from build123d import *

# Parameters (mm, degrees)
CORNERBOSS_EXTRUDE1_DEPTH               = 20
SHELL4_T                                = -3
PADSKETCH2_R                            = 12
PADBOSS_EXTRUDE2_DEPTH                  = 10
STEPPERSHAFTHOLECUTSKETCH3_R            = 5.1
STEPPERSHAFTHOLECUT_EXTRUDE1_DEPTH      = 288.430740571
THREADEDNUTMOUNTHOLESSKETCH4_R          = 2
THREADEDNUTMOUNTHOLESCUT_EXTRUDE2_DEPTH = 10
BRPEGHOLESKETCH1_W                      = 10
BRPEGHOLESKETCH1_H                      = 14
BRPEGHOLECUT_EXTRUDE1_DEPTH             = 3
TOPPEGSKETCH2_W                         = 9.8
TOPPEGSKETCH2_H                         = 13.9
TOPPEGBOSS_EXTRUDE1_DEPTH               = 3
TOPPEGCAPSKETCH3_W                      = 16
TOPPEGCAPSKETCH3_H                      = 17
TOPPEGCAPBOSS_EXTRUDE2_DEPTH            = 3.1
CENTERPEGHOLECUTSKETCH1_W               = 10
CENTERPEGHOLECUTSKETCH1_H               = 14
CENTERPEGHOLECUT_EXTRUDE1_DEPTH         = 3


with BuildPart() as part:
    # CornerrSketch1 → CornerBoss-Extrude1 (new body)
    with BuildSketch(Plane(origin=(0, 0, 0), x_dir=(1, 0, 0), z_dir=(0, 1, 0))):
        with BuildLine():
            Line((0, 195.825), (70, 195.825))
            Line((70, 195.825), (70, 125.825))
            Line((70, 125.825), (210, 125.825))
            Line((210, 125.825), (210, 45.825))
            Line((210, 45.825), (34, 45.825))
            Line((34, 45.825), (34, 0))
            ThreePointArc((34, 0), (17, -17), (0, 0))
            Line((0, 0), (0, 195.825))
        make_face()
    extrude(amount=CORNERBOSS_EXTRUDE1_DEPTH)

    # Shell4
    shell4_openings = [part.faces().sort_by_distance(p)[0] for p in [
        (83.067785517, 0, -95.408443826),
    ]]
    offset(amount=SHELL4_T, openings=shell4_openings, kind=Kind.INTERSECTION)

    # PadSketch2 → PadBoss-Extrude2 (add)
    with BuildSketch(Plane.XZ.offset(-17)):
        with Locations(Location((17, 0, 0), (0, 0, 90))):
            Circle(PADSKETCH2_R)
    extrude(amount=PADBOSS_EXTRUDE2_DEPTH)

    # StepperShaftHoleCutSketch3 → StepperShaftHoleCut-Extrude1 (cut, through all)
    with BuildSketch(Plane.XZ.offset(-7)):
        with Locations(Location((17, 0, 0), (0, 0, 270))):
            Circle(STEPPERSHAFTHOLECUTSKETCH3_R)
    extrude(amount=-STEPPERSHAFTHOLECUT_EXTRUDE1_DEPTH, mode=Mode.SUBTRACT)

    # ThreadedNutMountHolesSketch4 → ThreadedNutMountHolesCut-Extrude2 (cut)
    with BuildSketch(Plane(origin=(0, 7, 0), x_dir=(-1, 0, 0), z_dir=(0, -1, 0))):
        with Locations(Location((-17, 8, 0), (0, 0, 90))):
            Circle(THREADEDNUTMOUNTHOLESSKETCH4_R)
        with Locations(Location((-17, -8, 0), (0, 0, 90))):
            Circle(THREADEDNUTMOUNTHOLESSKETCH4_R)
        with Locations(Location((-25, 0, 0), (0, 0, 90))):
            Circle(THREADEDNUTMOUNTHOLESSKETCH4_R)
        with Locations(Location((-9, 0, 0), (0, 0, 90))):
            Circle(THREADEDNUTMOUNTHOLESSKETCH4_R)
    extrude(amount=-THREADEDNUTMOUNTHOLESCUT_EXTRUDE2_DEPTH, mode=Mode.SUBTRACT)

    # BRPegHoleSketch1 → BRPegHoleCut-Extrude1 (cut)
    with BuildSketch(Plane(origin=(210, 0, 0), x_dir=(0, 0, -1), z_dir=(1, 0, 0))):
        with Locations((60.825, 7)):
            Rectangle(BRPEGHOLESKETCH1_W, BRPEGHOLESKETCH1_H)
    extrude(amount=-BRPEGHOLECUT_EXTRUDE1_DEPTH, mode=Mode.SUBTRACT)

    # TopPegSketch2 → TopPegBoss-Extrude1 (add)
    with BuildSketch(Plane(origin=(0, 0, -195.825), x_dir=(-1, 0, 0), z_dir=(0, 0, -1))):
        with Locations((-15, 6.95)):
            Rectangle(TOPPEGSKETCH2_W, TOPPEGSKETCH2_H)
    extrude(amount=TOPPEGBOSS_EXTRUDE1_DEPTH)

    # TopPegCapSketch3 → TopPegCapBoss-Extrude2 (add)
    with BuildSketch(Plane(origin=(0, 0, -198.825), x_dir=(-1, 0, 0), z_dir=(0, 0, -1))):
        with Locations((-14.9, 8.5)):
            Rectangle(TOPPEGCAPSKETCH3_W, TOPPEGCAPSKETCH3_H)
    extrude(amount=TOPPEGCAPBOSS_EXTRUDE2_DEPTH)

    # CenterPegHoleCutSketch1 → CenterPegHoleCut-Extrude1 (cut)
    with BuildSketch(Plane(origin=(0, 0, -125.825), x_dir=(-1, 0, 0), z_dir=(0, 0, -1))):
        with Locations((-175, 7)):
            Rectangle(CENTERPEGHOLECUTSKETCH1_W, CENTERPEGHOLECUTSKETCH1_H)
    extrude(amount=-CENTERPEGHOLECUT_EXTRUDE1_DEPTH, mode=Mode.SUBTRACT)


solid = part.part
Design review of the part built by this model. Coordinates are the model's own, in mm. A direction names the side the tool comes from. Coordinates: 2 decimals unless noted, no trailing zeros. Write each loop counter-clockwise with the first axis right and the second up, starting at its lowest first coordinate (ties: lowest second). Pieces come first, ordered by that corner, then holes. Notation, with made-up numbers: (-17, -16) - (35, -16) arc R28 cw to (35, 11) - close; hole circle Ø4 at (-38, -15). An arc over 180 degrees is marked (long way). One line per item, written item: value.
1) Add section B-B (y = 10.5). Give the number of separate pieces and of enclosed holes in the cut face, plus the area to 3 significant figures.
Answer sheet:
separate pieces: 3
enclosed holes: 5
area: 2,800 mm2
2) Insertion check: pin 1 (1.5 mm diameter, centred on y = 8, z = -197, fed in from +X); pin 2 (4 mm diameter, centred on y = 12.5, z = -8, fed in from +X); pin 3 (1.2 mm diameter, centred on x = 26, z = 0, fed in from -Y). Each pin has a flat end and moves straight along its axis. Give the tip position at first contact, or say it passes through.
Answer sheet:
pin 1: stops at x = 19.9
pin 2: stops at x = 34
pin 3: stops at y = 17
3) Mouldability with a two-part tool opening along Z and no side actions: class faces 1 (the face through (35, 8, -192.825)), 2 (the face through (123, 10, -45.825)), 3 (the face through (120, 8, -48.825)), 4 (the face through (105, 0, -124)) as +Z half, -Z half, draft (parallel to the pull), parting line (faces both ways), or undercut.
Answer sheet:
face 1: undercut
face 2: +Z half
face 3: undercut
face 4: draft
4) Add section A-A (x = 47.5). State the section outline as (y, z) points (3 decimals), plus the area to 3 significant figures.
Answer sheet:
outline: (0, -195.825) - (20, -195.825) - (20, -45.825) - (0, -45.825) - (0, -48.825) - (17, -48.825) - (17, -192.825) - (0, -192.825) - close
area: 552 mm2
5) For faces 5 (the face through (34, 10, -23)), 6 (the face through (15, 14.3, -198.825)), 7 (the face through (70, 10, -161)), 8 (the face through (31, 8, -25)), list the 3-axis set-ups (+Z, -Z, +X, -X, +Y, -Y) from which the entire face can be reached by the end or side of a thin tool; tool diameter is ignored.
Answer sheet:
face 5: +Z, +X, +Y, -Y
face 6: +Y
face 7: -Z, +X, +Y, -Y
face 8: -Y
6) Add section C-C (z = -92). State the section outline as (x, y) points, plus the area to 3 significant figures.
Answer sheet:
outline: (0, 0) - (3, 0) - (3, 17) - (207, 17) - (207, 0) - (210, 0) - (210, 20) - (0, 20) - close
area: 732 mm2
7) To check wall thickness, follow probe 1 along X at (y, z) = (10, 0); probe 2 along Z at (x, y) = (51, 11.25) (3 decimals); probe 3 along X at (y, z) = (14, -111.5). State the ranges of each line that lie inside material, in increasing order.
Answer sheet:
probe 1: x = 0 to 3, 5 to 7, 11 to 11.9, 22.1 to 23, 27 to 29, 31 to 34
probe 2: z = -195.825 to -192.825, -48.825 to -45.825
probe 3: x = 0 to 3, 207 to 210
